Here's how the part is built. I have some questions about the finished solid (model axes, mm). A direction names the side the tool comes from. Give positions to 0.01 mm unless a question says otherwise; leave off trailing zeros. Order: outer loops, then holes, each group sorted by start corner. A loop starts at its lowest first (then second) coordinate and runs counter-clockwise, first axis right, second up.
from build123d import *

# Parameters (mm, degrees)
SKETCH1_W           = 44.45
SKETCH1_H           = 53.975
BOSS_EXTRUDE1_DEPTH = 3.175
SKETCH2_W           = 31.75
SKETCH2_H           = 3.175
CUT_EXTRUDE1_DEPTH  = 4.175
SKETCH3_R           = 1.5875
SKETCH3_R_2         = 1.1
SKETCH3_W           = 12.7
SKETCH3_H           = 6.35
SKETCH3_W_2         = 25.4
SKETCH3_H_2         = 7.62
CUT_EXTRUDE2_DEPTH  = 4.175


with BuildPart() as part:
    # Sketch1 → Boss-Extrude1 (new body)
    with BuildSketch(Plane.XY):
        with Locations((22.225, 26.9875)):
            Rectangle(SKETCH1_W, SKETCH1_H)
    extrude(amount=BOSS_EXTRUDE1_DEPTH)

    # Sketch2 → Cut-Extrude1 (cut, through all)
    with BuildSketch(Plane.XY.offset(3.175)):
        with Locations((22.225, 1.5875)):
            Rectangle(SKETCH2_W, SKETCH2_H)
    extrude(amount=-CUT_EXTRUDE1_DEPTH, mode=Mode.SUBTRACT)

    # Sketch3 → Cut-Extrude2 (cut, through all)
    with BuildSketch(Plane.XY.offset(3.175)):
        with Locations((3.81, 20.955)):
            Circle(SKETCH3_R)
        with Locations((40.64, 20.955)):
            Circle(SKETCH3_R)
        with Locations((11.677212596, 47.625)):
            Circle(SKETCH3_R_2)
        with Locations((11.677212596, 33.325)):
            Circle(SKETCH3_R_2)
        with Locations((32.677212596, 47.625)):
            Circle(SKETCH3_R_2)
        with Locations((32.677212596, 33.325)):
            Circle(SKETCH3_R_2)
        with Locations((22.225, 6.35)):
            Rectangle(SKETCH3_W, SKETCH3_H)
        with Locations((22.225, 24.765)):
            Rectangle(SKETCH3_W_2, SKETCH3_H_2)
    extrude(amount=-CUT_EXTRUDE2_DEPTH, mode=Mode.SUBTRACT)


solid = part.part
Q1. If we section it at C-C on z = 2.3: Give the number of separate pieces and of enclosed holes in the cut face, plus the area to 3 significant figures.
Filled sheet:
separate pieces: 1
enclosed holes: 7
area: 1,990 mm2
Q2. I'm going to push flat-ended pins straight in: P1, Ø3, axis at x = 20.5, y = 40, coming from the -Z side; P2, Ø1.6, axis at x = 24.5, z = 1.5, coming from the -Y side (3 decimals). Where does each tip first touch, or does it pass through?
Filled sheet:
P1: stops at z = 0
P2: stops at y = 9.525
Q3. I need wall thicknesses on L1, parallel to Y at x = 11.5, z = 2.05 (3 decimals); L2, parallel to Y at x = 31, z = 1.05 (3 decimals); L3, parallel to Y at x = 18, z = 1.05 (3 decimals). Which ranges of each line are inside material? Lowest first, please.
Filled sheet:
L1: y = 3.175 to 20.955, 28.575 to 32.239, 34.411 to 46.539, 48.711 to 53.975
L2: y = 3.175 to 20.955, 28.575 to 53.975
L3: y = 9.525 to 20.955, 28.575 to 53.975
Q4. Thinking about a two-plate mould opening in X: for faces 4 (the face through (3, 0, 2)), 5 (the face through (44.45, 27, 2)), 6 (the face through (22, 9.525, 2)), which applies, released by +X, released by -X, zero draft, split by the parting line, or undercut?
Filled sheet:
face 4: zero draft
face 5: released by +X
face 6: undercut
Q5. If we section it at A-A on x = 40.64: List the corners of the cut face in (y, z) for me (1 decimal), plus the area to 3 significant figures.
Filled sheet:
outline: (0, 0) - (19.4, 0) - (19.4, 3.2) - (0, 3.2) - close; (22.5, 0) - (54, 0) - (54, 3.2) - (22.5, 3.2) - close
area: 161 mm2
Q6. For faces 1 (the face through (34.925, 25, 2)), 2 (the face through (28.575, 6, 2)), 3 (the face through (22, 33, 3.175)), which set-ups out of +Z, -Z, +X, -X, +Y, -Y let a thin tool reach every point of the face, with its end or its side?
Filled sheet:
face 1: +Z, -Z
face 2: +Z, -Z, -Y
face 3: +Z, +X, -X, +Y, -Y
Q7. If we section it at B-B on y = 5: List the corners of the cut face in (x, z) for me (3 decimals).
Filled sheet:
outline: (0, 0) - (15.875, 0) - (15.875, 3.175) - (0, 3.175) - close; (28.575, 0) - (44.45, 0) - (44.45, 3.175) - (28.575, 3.175) - close
